Source: CAD feature listing. Evaluate the final solid. Frame: model axes, mm. A direction names the side the tool comes from. Round coordinates to 2 decimals unless told otherwise and drop trailing zeros. Write each loop counter-clockwise with the first axis right and the second up, starting at its lowest first coordinate (ties: lowest second). Pieces come first, ordered by that corner, then holes. Notation, with made-up numbers: M 46,37 L 89,37 A24 cw 89,66 Z; hole C 32.5,-39.75 d5. An arc over 180 degrees is marked long. Use a Markdown table: item, result.
```python
from build123d import *

# Parameters (mm, degrees)
CROQUIS1_W              = 15
CROQUIS1_H              = 19.98
SALIENTE_EXTRUIR1_DEPTH = 1.6
CROQUIS2_W              = 8.49
CROQUIS2_H              = 9.01
SALIENTE_EXTRUIR2_DEPTH = 6
CORTAR_EXTRUIR1_DEPTH   = 18.820847342
REDONDEO1_R             = 0.1
REDONDEO2_R             = 0.1


with BuildPart() as part:
    # Croquis1 → Saliente-Extruir1 (new body)
    with BuildSketch(Plane.XY):
        Rectangle(CROQUIS1_W, CROQUIS1_H)
    extrude(amount=SALIENTE_EXTRUIR1_DEPTH)

    # Croquis2 → Saliente-Extruir2 (add)
    with BuildSketch(Plane.XY.offset(1.6)):
        with Locations((-0.905, -0.015)):
            Rectangle(CROQUIS2_W, CROQUIS2_H)
    extrude(amount=SALIENTE_EXTRUIR2_DEPTH)

    # Croquis3 → Cortar-Extruir1 (cut, through all)
    with BuildSketch(Plane.ZY.offset(5.15)):
        with BuildLine():
            ThreePointArc((7.215, 3.45), (7.487236111, 3.337236111), (7.6, 3.065))
            Line((7.6, 3.065), (7.6, 4.49))
            ThreePointArc((7.6, 4.49), (7.441092235, 4.307099962), (7.215, 4.22))
            ThreePointArc((7.215, 4.22), (7.153028067, 4.216157783), (7.091056134, 4.22))
            Line((7.091056134, 4.22), (3.9, 4.22))
            ThreePointArc((3.9, 4.22), (3.6659049, 4.14065419), (3.528300528, 3.935321996))
            Line((3.528300528, 3.935321996), (3.528300528, 3.734678004))
            ThreePointArc((3.528300528, 3.734678004), (3.6659049, 3.52934581), (3.9, 3.45))
            Line((3.9, 3.45), (7.215, 3.45))
        make_face()
        with BuildLine():
            ThreePointArc((7.215, 1.91), (7.487236111, 1.797236111), (7.6, 1.525))
            Line((7.6, 1.525), (7.6, 3.065))
            ThreePointArc((7.6, 3.065), (7.487236111, 2.792763889), (7.215, 2.68))
            Line((7.215, 2.68), (3.9, 2.68))
            ThreePointArc((3.9, 2.68), (3.6659049, 2.60065419), (3.528300528, 2.395321996))
            Line((3.528300528, 2.395321996), (3.528300528, 2.194678004))
            ThreePointArc((3.528300528, 2.194678004), (3.6659049, 1.98934581), (3.9, 1.91))
            Line((3.9, 1.91), (7.215, 1.91))
        make_face()
        with BuildLine():
            Line((3.9, 0.37), (7.215, 0.37))
            ThreePointArc((7.215, 0.37), (7.487236111, 0.257236111), (7.6, -0.015))
            Line((7.6, -0.015), (7.6, 1.525))
            ThreePointArc((7.6, 1.525), (7.487236111, 1.252763889), (7.215, 1.14))
            Line((7.215, 1.14), (3.9, 1.14))
            ThreePointArc((3.9, 1.14), (3.6659049, 1.06065419), (3.528300528, 0.855321996))
            Line((3.528300528, 0.855321996), (3.528300528, 0.654678004))
            ThreePointArc((3.528300528, 0.654678004), (3.6659049, 0.44934581), (3.9, 0.37))
        make_face()
        with BuildLine():
            Line((7.6, -1.555), (7.6, -0.015))
            ThreePointArc((7.6, -0.015), (7.487236111, -0.287236111), (7.215, -0.4))
            Line((7.215, -0.4), (3.9, -0.4))
            ThreePointArc((3.9, -0.4), (3.6659049, -0.47934581), (3.528300528, -0.684678004))
            Line((3.528300528, -0.684678004), (3.528300528, -0.885321996))
            ThreePointArc((3.528300528, -0.885321996), (3.6659049, -1.09065419), (3.9, -1.17))
            Line((3.9, -1.17), (7.215, -1.17))
            ThreePointArc((7.215, -1.17), (7.487236111, -1.282763889), (7.6, -1.555))
        make_face()
        with BuildLine():
            Line((7.6, -3.095), (7.6, -1.555))
            ThreePointArc((7.6, -1.555), (7.487236111, -1.827236111), (7.215, -1.94))
            Line((7.215, -1.94), (3.9, -1.94))
            ThreePointArc((3.9, -1.94), (3.6659049, -2.01934581), (3.528300528, -2.224678004))
            Line((3.528300528, -2.224678004), (3.528300528, -2.425321996))
            ThreePointArc((3.528300528, -2.425321996), (3.6659049, -2.63065419), (3.9, -2.71))
            Line((3.9, -2.71), (7.215, -2.71))
            ThreePointArc((7.215, -2.71), (7.487236111, -2.822763889), (7.6, -3.095))
        make_face()
        with BuildLine():
            Line((7.6, -4.52), (7.6, -3.095))
            ThreePointArc((7.6, -3.095), (7.487236111, -3.367236111), (7.215, -3.48))
            Line((7.215, -3.48), (3.9, -3.48))
            ThreePointArc((3.9, -3.48), (3.6659049, -3.55934581), (3.528300528, -3.764678004))
            Line((3.528300528, -3.764678004), (3.528300528, -3.965321996))
            ThreePointArc((3.528300528, -3.965321996), (3.6659049, -4.17065419), (3.9, -4.25))
            Line((3.9, -4.25), (7.091056134, -4.25))
            ThreePointArc((7.091056134, -4.25), (7.153028067, -4.246157783), (7.215, -4.25))
            ThreePointArc((7.215, -4.25), (7.441092235, -4.337099962), (7.6, -4.52))
        make_face()
    extrude(amount=-CORTAR_EXTRUIR1_DEPTH, mode=Mode.SUBTRACT)

    # Redondeo1
    redondeo1_edges = [part.edges().sort_by_distance(p)[0] for p in [
        (-0.905, -4.52, 7.6),
    ]]
    fillet(redondeo1_edges, radius=REDONDEO1_R)

    # Redondeo2
    redondeo2_edges = [part.edges().sort_by_distance(p)[0] for p in [
        (-0.905, 4.49, 7.6),
    ]]
    fillet(redondeo2_edges, radius=REDONDEO2_R)


solid = part.part
```
Q1. Section A-A on z = 5.25. Return loops of the section in (x, y).
Results are:
| item | result |
|---|---|
| outline | M -5.15,-4.52 L 3.34,-4.52 L 3.34,-4.25 L -5.15,-4.25 Z; M -5.15,-3.48 L 3.34,-3.48 L 3.34,-2.71 L -5.15,-2.71 Z; M -5.15,-1.94 L 3.34,-1.94 L 3.34,-1.17 L -5.15,-1.17 Z; M -5.15,-0.4 L 3.34,-0.4 L 3.34,0.37 L -5.15,0.37 Z; M -5.15,1.14 L 3.34,1.14 L 3.34,1.91 L -5.15,1.91 Z; M -5.15,2.68 L 3.34,2.68 L 3.34,3.45 L -5.15,3.45 Z; M -5.15,4.22 L 3.34,4.22 L 3.34,4.49 L -5.15,4.49 Z |
Q2. Reachability of faces 1 (the flat face through (3.34, 0, 4)), 2 (the flat face through (-1, -4.52, 4)), 3 (the flat face through (-1, 3.45, 6)) from +Z, -Z, +X, -X, +Y, -Y: full face, straight path, thin tool, end or side. Return the list, or none.
Results are:
| item | result |
|---|---|
| face 1 | +Z, +X, +Y, -Y |
| face 2 | +Z, +X, -X, -Y |
| face 3 | +Z, +X, -X |
Q3. Mould query, pull axis Y, two halves, no side actions, for faces 4 (the flat face through (-1, 4.49, 4)), 5 (the flat face through (-5.15, 0, 4)), 6 (the flat face through (-1, -3.48, 6)). Classes: +Y half, -Y half, draft (parallel to the pull), parting line (faces both ways), or undercut.
Results are:
| item | result |
|---|---|
| face 4 | +Y half |
| face 5 | draft |
| face 6 | undercut |
Q4. Section B-B on y = -6.75. Return loops of the section in (x, z), plus the area to 3 significant figures.
Results are:
| item | result |
|---|---|
| outline | M -7.5,0 L 7.5,0 L 7.5,1.6 L -7.5,1.6 Z |
| area | 24.0 mm^2 |
Q5. Section C-C on x = 6. Return loops of the section in (y, z).
Results are:
| item | result |
|---|---|
| outline | M -9.99,0 L 9.99,0 L 9.99,1.6 L -9.99,1.6 Z |
Q6. First-contact query: pin 1 Ø1 at (y, z) = (-1, 6.5) entering from +X; pin 2 Ø3 at (x, z) = (1, 6) entering from +Y; pin 3 Ø2.5 at (x, z) = (-2, 6) entering from -Y. Flat tips, straight axial feed; report the tip coordinate or a pass-through.
Results are:
| item | result |
|---|---|
| pin 1 | x = 3.34 |
| pin 2 | y = 4.49 |
| pin 3 | y = -4.52 |
Q7. Line query: L1, parallel to Z at x = 2.5, y = 8.25; L2, parallel to X at y = 0.5, z = 2.5; L3, parallel to Y at x = 0.5, z = 2. Output: solid intervals per line, ascending.
Results are:
| item | result |
|---|---|
| L1 | 0 to 1.6 |
| L2 | -5.15 to 3.34 |
| L3 | -4.52 to 4.49 |
